from build123d import *

# Parameters (mm, degrees)
ESQUISSE1_W             = 50
ESQUISSE1_H             = 70
ESQUISSE1_R             = 10
BOSS_EXTRU_1_DEPTH      = 20
ESQUISSE2_W             = 50
ESQUISSE2_H             = 90
BOSS_EXTRU_2_DEPTH      = 20
ESQUISSE3_R             = 29.154759474
BOSS_EXTRU_3_DEPTH      = 20
ESQUISSE4_R             = 20
BOSS_EXTRU_4_DEPTH      = 75
ESQUISSE5_W             = 50
ESQUISSE5_H             = 20
BOSS_EXTRU_5_DEPTH      = 75
ESQUISSE6_R             = 10
ENL_V_MAT_EXTRU_1_DEPTH = 75


with BuildPart() as part:
    # Esquisse1 → Boss.-Extru.1 (new body)
    with BuildSketch(Plane.XY):
        with Locations((-270.845240526, -10)):
            Rectangle(ESQUISSE1_W, ESQUISSE1_H)
        with Locations((-270.845240526, 0)):
            Circle(ESQUISSE1_R, mode=Mode.SUBTRACT)
    extrude(amount=BOSS_EXTRU_1_DEPTH)

    # Esquisse2 → Boss.-Extru.2 (add)
    with BuildSketch(Plane.XZ.offset(45)):
        with Locations((-270.845240526, -25)):
            Rectangle(ESQUISSE2_W, ESQUISSE2_H)
    extrude(amount=BOSS_EXTRU_2_DEPTH)

    # Esquisse3 → Boss.-Extru.3 (add)
    with BuildSketch(Plane.XZ.offset(65)):
        with Locations(Location((-270.845240526, -25, 0), (0, 0, 30.963756532))):
            Circle(ESQUISSE3_R)
    extrude(amount=BOSS_EXTRU_3_DEPTH)

    # Esquisse4 → Boss.-Extru.4 (add)
    with BuildSketch(Plane.XZ.offset(85)):
        with Locations(Location((-270.845240526, -25, 0), (0, 0, 270))):
            Circle(ESQUISSE4_R)
    extrude(amount=BOSS_EXTRU_4_DEPTH)

    # Esquisse5 → Boss.-Extru.5 (add)
    with BuildSketch(Plane(origin=(0, -45, 0), x_dir=(1, 0, 0), z_dir=(0, 1, 0))):
        with Locations((-270.845240526, 60)):
            Rectangle(ESQUISSE5_W, ESQUISSE5_H)
    extrude(amount=BOSS_EXTRU_5_DEPTH)

    # Esquisse6 → Enlèv. mat.-Extru.1 (cut)
    with BuildSketch(Plane(origin=(0, 0, -70), x_dir=(-1, 0, 0), z_dir=(0, 0, -1))):
        with Locations(Location((270.845240526, 0, 0), (0, 0, 180))):
            Circle(ESQUISSE6_R)
    extrude(amount=-ENL_V_MAT_EXTRU_1_DEPTH, mode=Mode.SUBTRACT)


solid = part.part
CAD build for the part. Positions are in the model's coordinates, mm. A direction names the side the tool comes from. Round coordinates to 2 decimals unless told otherwise and drop trailing zeros. Write each loop counter-clockwise with the first axis right and the second up, starting at its lowest first coordinate (ties: lowest second). Pieces come first, ordered by that corner, then holes. Notation, with made-up numbers: (87, 83) -> (127, 83) arc R24 ccw to (127, 114) -> close; hole circle Ø7 at (26.25, 22). An arc over 180 degrees is marked (long way). Answer as a JSON object with one key per item and string values.
(1) Band-saw the part on C-C, the plane y = -34. List the corners of the cut face in (x, z).
Reported:
{"outline": "(-295.85, -70) -> (-245.85, -70) -> (-245.85, -50) -> (-295.85, -50) -> close; (-295.85, 0) -> (-245.85, 0) -> (-245.85, 20) -> (-295.85, 20) -> close"}
(2) Which spindle directions (+Z, -Z, +X, -X, +Y, -Y) get a long thin tool onto all of the face, cutting with end or side? Do faces 4 (the face through (-245.845, -50, -24)), 5 (the face through (-271, -45, -25)), 6 (the face through (-299.41, -74.86, -19.16)), 7 (the face through (-297, -65, -25)). Say none if no direction does.
Reported:
{"face 4": "+Z, -Z, +X, +Y", "face 5": "+X, -X, +Y", "face 6": "-Y", "face 7": "+Z, -Z, -X, +Y"}
(3) Band-saw the part on A-A, the plane y = 0. List the corners of the cut face in (x, z).
Reported:
{"outline": "(-295.85, -70) -> (-280.85, -70) -> (-280.85, -50) -> (-295.85, -50) -> close; (-295.85, 0) -> (-280.85, 0) -> (-280.85, 20) -> (-295.85, 20) -> close; (-260.85, -70) -> (-245.85, -70) -> (-245.85, -50) -> (-260.85, -50) -> close; (-260.85, 0) -> (-245.85, 0) -> (-245.85, 20) -> (-260.85, 20) -> close"}
(4) Probe probe 1 along Y at (x, z) = (-280.5, -41); probe 2 along Y at (x, z) = (-289, -59); probe 3 along Z at (x, y) = (-259.5, -37.5). List the from-to ranges inside material, lowest first. Write a range as [from, to].
Reported:
{"probe 1": "y = [-160, -45]", "probe 2": "y = [-65, 30]", "probe 3": "z = [-70, -50], [0, 20]"}
(5) Band-saw the part on D-D, the plane x = -267. List the corners of the cut face in (y, z), then the cut area to 3 significant figures.
Reported:
{"outline": "(-160, -44.63) -> (-85, -44.63) -> (-85, -53.9) -> (-65, -53.9) -> (-65, -70) -> (-9.23, -70) -> (-9.23, -50) -> (-45, -50) -> (-45, 0) -> (-9.23, 0) -> (-9.23, 20) -> (-65, 20) -> (-65, 3.9) -> (-85, 3.9) -> (-85, -5.37) -> (-160, -5.37) -> close; (9.23, -70) -> (30, -70) -> (30, -50) -> (9.23, -50) -> close; (9.23, 0) -> (25, 0) -> (25, 20) -> (9.23, 20) -> close", "area": "8,060 mm^2"}
(6) Band-saw the part on B-B, the plane z = -63.5. List the corners of the cut face in (x, y).
Reported:
{"outline": "(-295.85, -65) -> (-245.85, -65) -> (-245.85, 30) -> (-295.85, 30) -> close; hole circle Ø20 at (-270.85, 0)"}
(7) Two-plate mould, pull along X, no slides. Class faces 1 (the face through (-271, 25, 10)), 2 (the face through (-261.307, 3.004, 9.86)), 3 (the face through (-251.015, -121.975, -22.396)): +X half, -X half, draft (parallel to the pull), parting line (faces both ways), or undercut.
Reported:
{"face 1": "draft", "face 2": "undercut", "face 3": "parting line"}
(8) Pin check, flat tips, straight feed: P1, Ø15, axis at x = -276.5, z = -21, coming from the +Y side; P2, Ø4, axis at y = -24.5, z = 10.5, coming from the -X side; P3, Ø1.2, axis at x = -243.5, z = -27, coming from the +Y side; P4, Ø12, axis at x = -270.85, y = 0, coming from the +Z side. Stop position of each tip, or through.
Reported:
{"P1": "stops at y = -45", "P2": "stops at x = -295.85", "P3": "stops at y = -65", "P4": "passes through"}
